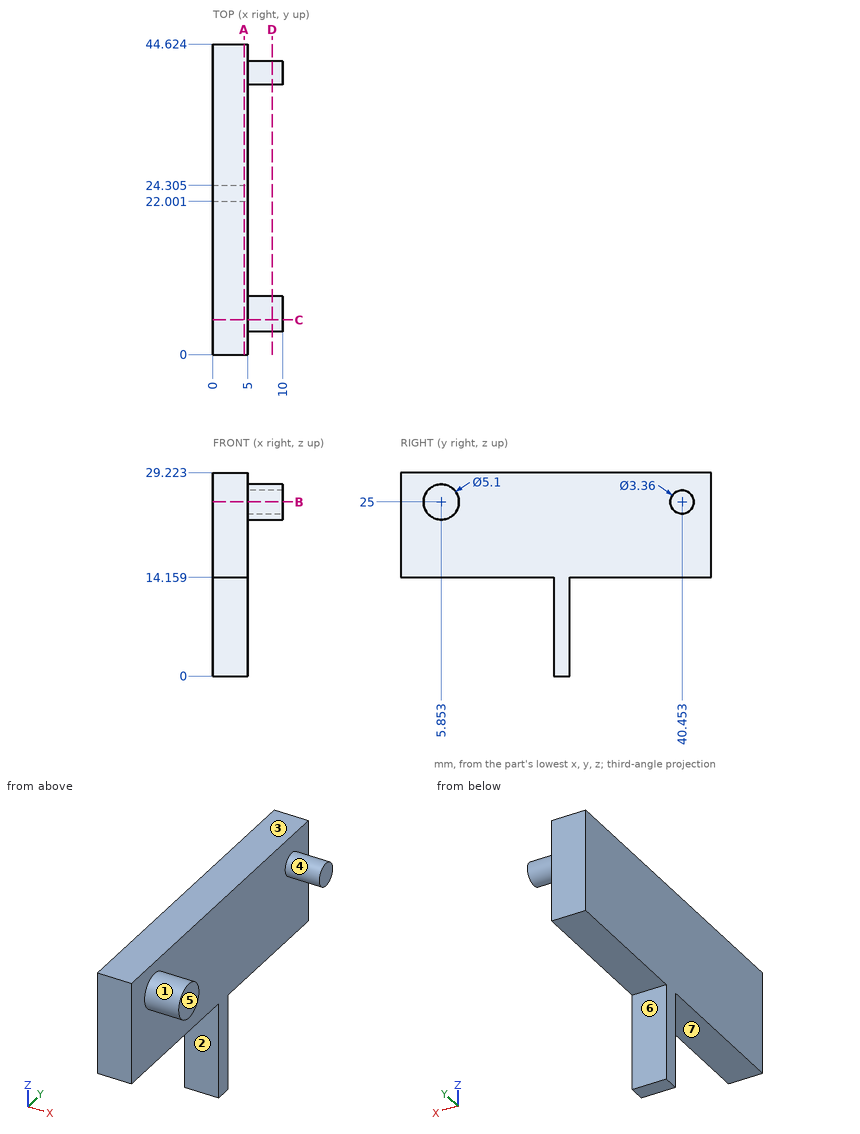
Could you check a few things on this drawing? It's one solid part, dimensions in mm from its lowest x, y, z. A direction names the side the tool comes from. Round coordinates to 2 decimals unless told otherwise and drop trailing zeros. Write each loop counter-clockwise with the first axis right and the second up, starting at its lowest first coordinate (ties: lowest second). Pieces come first, ordered by that corner, then holes. Notation, with made-up numbers: (66.25, 83.5) -> (108.25, 83.5) arc R19 cw to (108.25, 118.5) -> close; hole circle Ø10 at (45.5, 60). An arc over 180 degrees is marked (long way). One line per question, with ' | ' between items. Start each with the question number.
1) I'm going to push flat-ended pins straight in: P1, Ø4, axis at x = 5.5, y = 30, coming from the +Z side; P2, Ø4, axis at x = 3, y = 8, coming from the -Z side; P3, Ø4, axis at x = 1.5, z = 4.5, coming from the -Y side; P4, Ø1, axis at y = 5, z = 18.5, coming from the +X side. Where does each tip first touch, or does it pass through?
2) If we mould it in two halves opening along Y, with no side actions, what happens to the marked faces 1, 2, 3 and 4? For each: released by +Y, released by -Y, zero draft, split by the parting line, or undercut.
3) Suppose I cut it at B-B on z = 25. Write out the boundary of the cut face in (x, y) (1 decimal).
4) Suppose I cut it at A-A on x = 4.5. Write out the boundary of the cut face in (y, z) (1 decimal), then the cut area to 3 significant figures.
5) I need wall thicknesses on line 1 (Y direction, x = 4.75, z = 2) (1 decimal); line 2 (Z direction, x = 2.5, y = 8.5); line 3 (Z direction, x = 6.25, y = 5). Which ranges of each line are inside material? Lowest first, please. Write a range as [from, to].
6) On a 3-axis mill with a long thin cutter (end or side, diameter ignored), from which of +Z, -Z, +X, -X, +Y, -Y can I reach the whole of each face in a straight line? I mean the marked faces 5, 6 and 7. Say none if no direction works.
7) Suppose I cut it at D-D on x = 8.5. Write out the boundary of the cut face in (y, z).
8) Suppose I cut it at C-C on y = 5. Write out the boundary of the cut face in (x, z).
Return value:
1) P1: stops at z = 29.22 | P2: stops at z = 14.16 | P3: stops at y = 22 | P4: stops at x = 5
2) face 1: undercut | face 2: released by -Y | face 3: zero draft | face 4: undercut
3) outline: (0, 0) -> (5, 0) -> (5, 3.3) -> (10, 3.3) -> (10, 8.4) -> (5, 8.4) -> (5, 38.8) -> (10, 38.8) -> (10, 42.1) -> (5, 42.1) -> (5, 44.6) -> (0, 44.6) -> close
4) outline: (0, 14.2) -> (22, 14.2) -> (22, 0) -> (24.3, 0) -> (24.3, 14.2) -> (44.6, 14.2) -> (44.6, 29.2) -> (0, 29.2) -> close | area: 705 mm2
5) line 1: y = [22, 24.3] | line 2: z = [14.16, 29.22] | line 3: z = [22.6, 27.4]
6) face 5: +Z, -Z, +X, +Y, -Y | face 6: -Z, +X, -X, +Y | face 7: -Z, +X, -X, -Y
7) outline: circle Ø5.1 at (5.85, 25); circle Ø3.36 at (40.45, 25)
8) outline: (0, 14.16) -> (5, 14.16) -> (5, 22.6) -> (10, 22.6) -> (10, 27.4) -> (5, 27.4) -> (5, 29.22) -> (0, 29.22) -> close
